Here's how the part is built. I have some questions about the finished solid (model axes, mm). Give positions to 0.01 mm unless a question says otherwise; leave off trailing zeros. Write each loop counter-clockwise with the first axis right and the second up, starting at its lowest first coordinate (ties: lowest second). Pieces come first, ordered by that corner, then holes. Notation, with made-up numbers: (22, 71.5) -> (49, 71.5) arc R29 cw to (49, 93.5) -> close; hole circle Ø9 at (-8, 19). An arc over 180 degrees is marked (long way). Use one line per item in the form item = value.
```python
from build123d import *

# Parameters (mm, degrees)
RESSALTO_EXTRUS_O1_DEPTH = 50
FILETE1_R                = 0.25


with BuildPart() as part:
    # Esboço1 → Ressalto-extrusão1 (new, symmetric)
    with BuildSketch(Plane(origin=(0, 0, -50), x_dir=(-1, 0, 0), z_dir=(0, 0, -1))):
        Polygon((0.75, -1.299038106), (1.5, 0), (0.75, 1.299038106), (-0.75, 1.299038106), (-1.5, 0), (-0.75, -1.299038106), align=None)
    extrude(amount=RESSALTO_EXTRUS_O1_DEPTH, both=True)

    # Filete1
    filete1_edges = [part.edges().sort_by_distance(p)[0] for p in [
        (-1.125, 0.649519053, 0),
        (0, 1.299038106, 0),
        (1.125, 0.649519053, 0),
        (1.125, -0.649519053, 0),
        (0, -1.299038106, 0),
        (1.125, -0.649519053, -100),
        (1.125, 0.649519053, -100),
        (0, 1.299038106, -100),
        (-1.125, -0.649519053, 0),
        (-1.125, 0.649519053, -100),
        (-1.125, -0.649519053, -100),
        (0, -1.299038106, -100),
    ]]
    fillet(filete1_edges, radius=FILETE1_R)


solid = part.part
```
Q1. If I drill on line 1 along Y through (x, z) = (-0.8, -55.5); line 2 along X through (y, z) = (-0.8, -73.5); line 3 along Z through (x, y) = (-1.05, -0.4), over which ranges is the centre line in solid material (lowest first)? Write a range as from..to.
Result set:
line_1 = -1.21..1.21
line_2 = -1.04..1.04
line_3 = -99.99..-0.01
Q2. Will this pin go through, and if not, where does the flat tip stop? pin 1 Ø1 at (y, z) = (-1, -24) entering from +X.
Result set:
pin_1 = 1.21
Q3. If we mould it in two halves opening along Z, with no side actions, what happens to faces 1 (the face through (0, 0, -100)), 2 (the face through (0, 0, 0))? For each: +Z half, -Z half, draft (parallel to the pull), parting line (faces both ways), or undercut.
Result set:
face_1 = -Z half
face_2 = +Z half
Q4. I want a section at A-A, the plane z = -77. Write out the boundary of the cut face in (x, y), and give its area (3 significant figures).
Result set:
outline = (-1.5, 0) -> (-0.75, -1.3) -> (0.75, -1.3) -> (1.5, 0) -> (0.75, 1.3) -> (-0.75, 1.3) -> close
area = 5.85 mm2
